Read the model definition and answer for the solid it produces. Units are mm, in the model's axes. A direction names the side the tool comes from. Give positions to 0.01 mm unless a question says otherwise; leave off trailing zeros. Order: outer loops, then holes, each group sorted by start corner. A loop starts at its lowest first (then second) coordinate and runs counter-clockwise, first axis right, second up. Notation, with made-up numbers: (28.5, 42.5) - (61.5, 42.5) arc R21 ccw to (61.5, 59.5) - close; hole circle Ø7 at (-5, 14). An arc over 180 degrees is marked (long way). Return JSON: item names as keys, results as strings.
Autodesk Inventor part; units mm, degrees
ref_plane "YZ Plane" through (0, 0, 0) normal (1, 0, 0) x (0, 1, 0)
ref_plane "XZ Plane" through (0, 0, 0) normal (0, 1, 0) x (-1, 0, 0)
ref_plane "XY Plane" through (0, 0, 0) normal (0, 0, 1) x (1, 0, 0)
sketch "Sketch1" plane through (0, 0, 0) normal (1, 0, 0) x (0, 1, 0)
  line L0 (0, 0) -> (177.8, 0)
  line L1 (177.8, 0) -> (177.8, -381)
  line L2 (177.8, -381) -> (0, -381)
  line L3 (0, -381) -> (0, 0)
  line L4 (3.175, 0) -> (174.625, 0)
  line L5 (174.625, 0) -> (174.625, -381)
  line L6 (174.625, -381) -> (3.175, -381)
  line L7 (3.175, -381) -> (3.175, 0)
  line L8 (177.8, -381) -> (0, -381)
  line L9 (0, -381) -> (0, -374.65)
  line L10 (0, -374.65) -> (177.8, -374.65)
  line L11 (177.8, -374.65) -> (177.8, -381)
  dimension "d0" = 177.8
  dimension "d1" = 381
  dimension "d2" = 171.45
  dimension "d3" = 381
  dimension "d4" = 0
  dimension "d5" = 3.175
  dimension "d10" = 6.35
extrude "Extrusion1" add sketch "Sketch1" along normal blind 3.175 contours L0 L5 L10 L7 | L10 L5 L2 L7
extrude "Extrusion2" add sketch "Sketch1" along normal blind 12.7 contours L0 L7 L10 L3 | L10 L7 L2 L3 | L0 L1 L10 L5 | L10 L1 L2 L5
extrude "Extrusion3" add sketch "Sketch1" along normal blind 12.7 contours L10 L7 L2 L3 | L10 L5 L2 L7 | L10 L1 L2 L5
sketch "Sketch2" plane through (3.175, 174.625, 0) normal (0, -1, 0) x (1, 0, 0)
  line L0 (0, 0) -> (0, -374.65)
  line L1 (0, 0) -> (0, -368.3)
  line L2 (0, 0) -> (368.3, 0) construction
  line L3 (0, -368.3) -> (0, -348.742)
  line L4 (0, -368.3) -> (4.7625, -368.3)
  line L5 (9.525, -381) -> (9.525, 0)
  line L6 (0, -348.742) -> (4.7625, -348.742)
  point P0 (-3.175, 0)
  dimension "d13" = 368.3
  dimension "d14" = 90
  dimension "d15" = 19.558
  dimension "d16" = 4.7625
hole "Hole1" at (7.9375, 174.625, -368.3) at (7.9375, 174.625, -348.742) direction (0, 1, 0) diameter 3.175 depth 25.4 tip angle 118
properties part number "glifPlate"
Q1. A cutting plane is placed at B-B (y = 152.5). Write down the section's boundary in (x, z) (3 decimals).
Values:
{"outline": "(0, -381) - (12.7, -381) - (12.7, -374.65) - (3.175, -374.65) - (3.175, 0) - (0, 0) - close"}
Q2. A cutting plane is placed at A-A (z = -313). Write down the section's boundary in (x, y) (3 decimals).
Values:
{"outline": "(0, 0) - (12.7, 0) - (12.7, 3.175) - (3.175, 3.175) - (3.175, 174.625) - (12.7, 174.625) - (12.7, 177.8) - (0, 177.8) - close"}
Q3. Consider L1, parallel to Y at x = 3.5, z = -49 (3 decimals); L2, parallel to Z at x = 5.25, y = 152; L3, parallel to X at y = 84, z = -365 (3 decimals). Determine where each line is inside the solid, lowest interval first.
Values:
{"L1": "y = 0 to 3.175, 174.625 to 177.8", "L2": "z = -381 to -374.65", "L3": "x = 0 to 3.175"}
Q4. Determine the mould class of faces 3 (the flat face through (8, 174.625, -185)), 4 (the flat face through (6, 0, -193)), 5 (the flat face through (6, 177.8, -188)), 6 (the flat face through (12.7, 3, -190)) for opening direction Y: released by +Y, released by -Y, zero draft, split by the parting line, or undercut.
Values:
{"face 3": "undercut", "face 4": "released by -Y", "face 5": "released by +Y", "face 6": "zero draft"}
Q5. Given pin 1 (8 mm diameter, centred on y = 98.5, z = -118.5, fed in from +X) (3 decimals), flat-ended and moving along its own axis, determine where the tip first touches the part or whether it passes through.
Values:
{"pin 1": "stops at x = 3.175"}
Q6. For faces 1 (the flat face through (8, 88, -374.65)), 2 (the flat face through (0, 88, -188)), determine the directions among +Z, -Z, +X, -X, +Y, -Y from which every point of the face is accessible in a straight line to the end or side of a thin tool.
Values:
{"face 1": "+Z, +X", "face 2": "+Z, -Z, -X, +Y, -Y"}
